Design review of the part built by this model. Coordinates are the model's own, in mm. Face numbers are marked on the shaded views. A direction names the side the tool comes from. Give positions to 0.01 mm unless a question says otherwise; leave off trailing zeros. Write each loop counter-clockwise with the first axis right and the second up, starting at its lowest first coordinate (ties: lowest second). Pieces come first, ordered by that corner, then holes. Notation, with made-up numbers: (87.25, 50) -> (127.25, 50) arc R6 ccw to (127.25, 55) -> close; hole circle Ø1 at (-27, 45.5). An arc over 180 degrees is marked (long way). Answer as a JSON object with one key per item and string values.
```python
from build123d import *

# Parameters (mm, degrees)
SKETCH1_R                    = 3.25
BASE_FLANGE1_DEPTH           = 3.175
EDGE_FLANGE1_STRIP_W         = 15.24
EDGE_FLANGE1_STRIP_H         = 3.175
EDGE_FLANGE1_STRIP_CUT_DEPTH = 18
EDGE_FLANGE1_DEPTH           = 18
EDGE_FLANGE2_STRIP_W         = 15.24
EDGE_FLANGE2_STRIP_H         = 3.175
EDGE_FLANGE2_STRIP_CUT_DEPTH = 18
EDGE_FLANGE2_DEPTH           = 18
SKETCH12_R                   = 4.125
BOSS_EXTRUDE1_DEPTH          = 3.175


# Sheet-metal steps are written as plain solids
with BuildPart() as part:
    # Sketch1 → Base-Flange1 (new body)
    with BuildSketch(Plane(origin=(0, 0, 0), x_dir=(1, 0, 0), z_dir=(0, 1, 0))):
        with BuildLine():
            Line((7, -5.5), (7, 10))
            Line((7, 10), (-11, 10))
            Line((-11, 10), (-11, -5.5))
            ThreePointArc((-11, -5.5), (-10.560660172, -6.560660172), (-9.5, -7))
            Line((-9.5, -7), (5.5, -7))
            ThreePointArc((5.5, -7), (6.560660172, -6.560660172), (7, -5.5))
        make_face()
        with Locations(Location((0, 0, 0), (0, 0, 270))):
            Circle(SKETCH1_R, mode=Mode.SUBTRACT)
    extrude(amount=-BASE_FLANGE1_DEPTH)

    # Edge-Flange1 strip (across the edge) → Edge-Flange1 strip cut (cut)
    with BuildSketch(Plane(origin=(7, 0, -10), x_dir=(0, 0, 1), z_dir=(-1, 0, 0))):
        with Locations((-6.35, -1.5875)):
            Rectangle(EDGE_FLANGE1_STRIP_W, EDGE_FLANGE1_STRIP_H)
    extrude(amount=EDGE_FLANGE1_STRIP_CUT_DEPTH, mode=Mode.SUBTRACT)

    # Edge-Flange1 section (across the edge) → Edge-Flange1 (add)
    with BuildSketch(Plane(origin=(7, 0, -10), x_dir=(0, 0, 1), z_dir=(-1, 0, 0))):
        with BuildLine():
            Line((-3.175, 1.27), (-3.175, 45.0625))
            Line((-3.175, 45.0625), (0, 45.0625))
            Line((0, 45.0625), (0, 1.27))
            ThreePointArc((0, 1.27), (0.371974388, 0.371974388), (1.27, 0))
            Line((1.27, 0), (1.27, -3.175))
            ThreePointArc((1.27, -3.175), (-1.873089642, -1.873089642), (-3.175, 1.27))
        make_face()
    extrude(amount=EDGE_FLANGE1_DEPTH)

    # Edge-Flange2 strip (across the edge) → Edge-Flange2 strip cut (cut)
    with BuildSketch(Plane(origin=(-11, 45.0625, -13.175), x_dir=(0, -1, 0), z_dir=(1, 0, 0))):
        with Locations((-6.35, -1.5875)):
            Rectangle(EDGE_FLANGE2_STRIP_W, EDGE_FLANGE2_STRIP_H)
    extrude(amount=EDGE_FLANGE2_STRIP_CUT_DEPTH, mode=Mode.SUBTRACT)

    # Edge-Flange2 section (across the edge) → Edge-Flange2 (add)
    with BuildSketch(Plane(origin=(-11, 45.0625, -13.175), x_dir=(0, -1, 0), z_dir=(1, 0, 0))):
        with BuildLine():
            Line((-3.175, 1.27), (-3.175, 3))
            Line((-3.175, 3), (0, 3))
            Line((0, 3), (0, 1.27))
            ThreePointArc((0, 1.27), (0.371974388, 0.371974388), (1.27, 0))
            Line((1.27, 0), (1.27, -3.175))
            ThreePointArc((1.27, -3.175), (-1.873089642, -1.873089642), (-3.175, 1.27))
        make_face()
    extrude(amount=EDGE_FLANGE2_DEPTH)

    # Sketch12 → Boss-Extrude1 (add)
    with BuildSketch(Plane(origin=(0, 48.2375, 0), x_dir=(1, 0, 0), z_dir=(0, 1, 0))):
        with BuildLine():
            Line((7, 16.175), (-11, 16.175))
            ThreePointArc((-11, 16.175), (-10.306151754, 23.403488178), (-8.249945193, 30.368004048))
            Line((-8.249945193, 30.368004048), (3.473693159, 59.484997741))
            ThreePointArc((3.473693159, 59.484997741), (7.760101436, 63.857301034), (13.882735104, 63.918037982))
            Line((13.882735104, 63.918037982), (15.737995377, 63.171037769))
            ThreePointArc((15.737995377, 63.171037769), (20.11029867, 58.884629492), (20.171035618, 52.761995824))
            Line((20.171035618, 52.761995824), (8.447397267, 23.64500213))
            ThreePointArc((8.447397267, 23.64500213), (7.365183288, 19.979467462), (7, 16.175))
        make_face()
        with Locations(Location((12.749994525, 55.749996676, 0), (0, 0, 270))):
            Circle(SKETCH12_R, mode=Mode.SUBTRACT)
    extrude(amount=-BOSS_EXTRUDE1_DEPTH)


solid = part.part
```
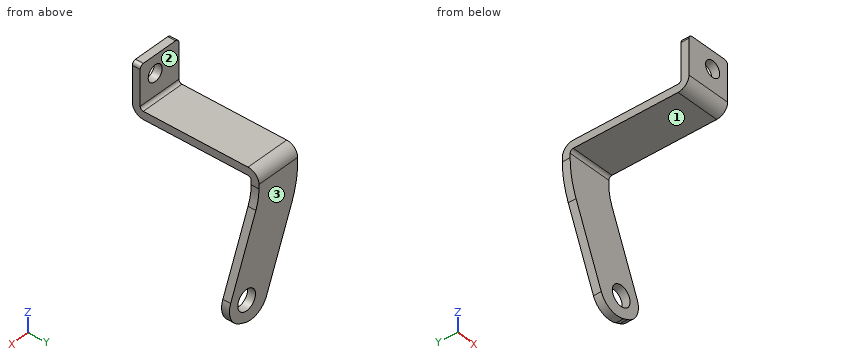
(1) We need section D-D, the plane x = -6.5. State the section outline as (y, z) points (1 decimal).
Here are the results:
{"outline": "(-3.2, -8.7) arc R4.4 ccw to (1.3, -13.2) -> (43.8, -13.2) arc R1.3 cw to (45.1, -14.4) -> (45.1, -34.7) -> (48.2, -34.7) -> (48.2, -14.4) arc R4.4 ccw to (43.8, -10) -> (1.3, -10) arc R1.3 cw to (0, -8.7) -> (0, 7) -> (-3.2, 7) -> close"}
(2) For the marked faces 1, 2 and 3, list the 3-axis set-ups (+Z, -Z, +X, -X, +Y, -Y) from which the entire face can be reached by the end or side of a thin tool; tool diameter is ignored.
Here are the results:
{"face 1": "-Z, +X, -X, -Y", "face 2": "+Z, +X, -X, +Y", "face 3": "+Z, -Z, +X, -X, +Y"}
(3) For line 1 along X through (y, z) = (-1.55, 0); line 2 along Z through (x, y) = (-8, 41.5) (3 decimals); line 3 along Y through (x, z) = (4, -16.5), list the stretches that pass through material, from the lowest coordinate up.
Here are the results:
{"line 1": "x = -11 to -3.25, 3.25 to 7", "line 2": "z = -13.175 to -10", "line 3": "y = 45.06 to 48.24"}
(4) We need section A-A, the plane z = 0. State the section outline as (x, y) points (3 decimals), then the cut area to 3 significant figures.
Here are the results:
{"outline": "(-11, -3.175) -> (-3.25, -3.175) -> (-3.25, 0) -> (-11, 0) -> close; (3.25, -3.175) -> (7, -3.175) -> (7, 0) -> (3.25, 0) -> close", "area": "36.5 mm²"}
(5) Clearance check with flat-ended pins moving along their axes: pin 1 (11 mm diameter, centred on y = 23.5, z = -5, fed in from +X); pin 2 (14.5 mm diameter, centred on x = 0.5, y = 12, fed in from -Z) (3 decimals); pin 3 (14.5 mm diameter, centred on x = -0.5, y = 18, fed in from +Z). State where each tip first meets the part, or that it passes through.
Here are the results:
{"pin 1": "stops at x = 7", "pin 2": "stops at z = -13.175", "pin 3": "stops at z = -10"}
(6) We need section C-C, the plane y = 22.5. State the section outline as (x, z) points (3 decimals).
Here are the results:
{"outline": "(-11, -13.175) -> (7, -13.175) -> (7, -10) -> (-11, -10) -> close"}
